Read the model definition and answer for the solid it produces. Units are mm, in the model's axes. Face numbers are marked on the shaded views. A direction names the side the tool comes from. Coordinates: 2 decimals unless noted, no trailing zeros. Write each loop counter-clockwise with the first axis right and the second up, starting at its lowest first coordinate (ties: lowest second). Pieces come first, ordered by that corner, then holes. Notation, with made-up numbers: (77, -3) - (113, -3) arc R24 ccw to (113, 29) - close; hole circle Ø9 at (85.25, -38). An arc over 180 degrees is marked (long way). Use a Markdown table: item, result.
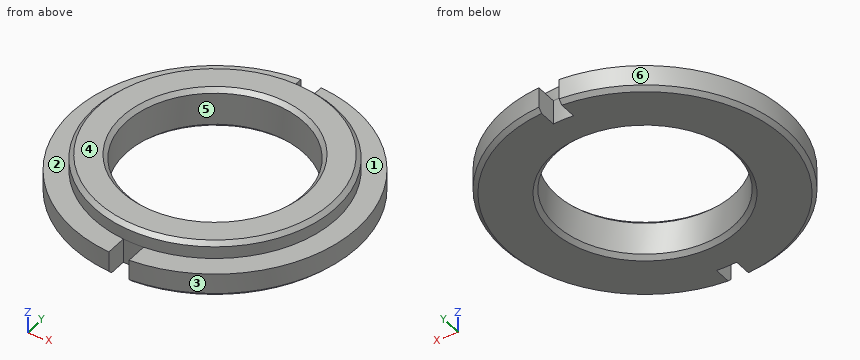
from build123d import *

# Parameters (mm, degrees)
SKETCH1_R           = 17.65
SKETCH1_R_2         = 11
BOSS_EXTRUDE1_DEPTH = 5
SKETCH2_R           = 17.65
SKETCH2_R_2         = 15
CUT_EXTRUDE1_DEPTH  = 2
CUT_EXTRUDE3_REACH  = 5
CHAMFER1_SIZE       = 0.5


with BuildPart() as part:
    # Sketch1 → Boss-Extrude1 (new body)
    with BuildSketch(Plane.XY):
        Circle(SKETCH1_R)
        Circle(SKETCH1_R_2, mode=Mode.SUBTRACT)
    extrude(amount=BOSS_EXTRUDE1_DEPTH)

    # Sketch2 → Cut-Extrude1 (cut)
    with BuildSketch(Plane.XY.offset(5)):
        Circle(SKETCH2_R)
        Circle(SKETCH2_R_2, mode=Mode.SUBTRACT)
    extrude(amount=-CUT_EXTRUDE1_DEPTH, mode=Mode.SUBTRACT)

    # Sketch3 → Cut-Extrude3 (cut, up to next)
    with BuildSketch(Plane.XY.offset(3), mode=Mode.PRIVATE) as cut_extrude3_sk1:
        with BuildLine():
            Line((1.25, 17.605680901), (1.25, 14.947825929))
            ThreePointArc((1.25, 14.947825929), (0, 15), (-1.25, 14.947825929))
            Line((-1.25, 14.947825929), (-1.25, 17.605680901))
            ThreePointArc((-1.25, 17.605680901), (0, 17.65), (1.25, 17.605680901))
        make_face()
    cut_extrude3_tool1 = extrude(cut_extrude3_sk1.sketch, amount=-CUT_EXTRUDE3_REACH, mode=Mode.PRIVATE) & part.part
    add(cut_extrude3_tool1.solids().sort_by_distance((0, 16.308915, 3))[0], mode=Mode.SUBTRACT)
    # Sketch3 → Cut-Extrude3 (cut, up to next)
    with BuildSketch(Plane.XY.offset(3), mode=Mode.PRIVATE) as cut_extrude3_sk2:
        with BuildLine():
            Line((1.25, -14.947825929), (1.25, -17.605680901))
            ThreePointArc((1.25, -17.605680901), (0, -17.65), (-1.25, -17.605680901))
            Line((-1.25, -17.605680901), (-1.25, -14.947825929))
            ThreePointArc((-1.25, -14.947825929), (0, -15), (1.25, -14.947825929))
        make_face()
    cut_extrude3_tool2 = extrude(cut_extrude3_sk2.sketch, amount=-CUT_EXTRUDE3_REACH, mode=Mode.PRIVATE) & part.part
    add(cut_extrude3_tool2.solids().sort_by_distance((0, -16.308915, 3))[0], mode=Mode.SUBTRACT)

    # Chamfer1
    chamfer1_edges = [part.edges().sort_by_distance(p)[0] for p in [
        (-15, 0, 5),
        (-17.65, 0, 0),
        (17.65, 0, 0),
        (-11, 0, 0),
        (-11, 0, 5),
    ]]
    chamfer(chamfer1_edges, length=CHAMFER1_SIZE)


solid = part.part
(1) The mould has two halves that part along Y. Classify the marked faces 4, 5 and 6: pulls with the +Y half, pulls with the -Y half, needs draft (parallel to the pull), parting line crosses it, or undercut.
Report:
| item | result |
|---|---|
| face 4 | needs draft |
| face 5 | undercut |
| face 6 | parting line crosses it |
(2) Each of these flat-tipped pins is pushed along its axis until it touches: P1, Ø3, axis at y = -3.5, z = 3.5, coming from the -X side; P2, Ø2, axis at x = 13, z = 1, coming from the -Y side; P3, Ø5, axis at x = 8.5, y = -6.5, coming from the +Z side; P4, Ø2, axis at y = 16.5, z = 1, coming from the -X side. Where does it stop, or does it pass through?
Report:
| item | result |
|---|---|
| P1 | stops at x = -17.53 |
| P2 | stops at y = -12.94 |
| P3 | stops at z = 5 |
| P4 | stops at x = -8.44 |
(3) A cutting plane is placed at A-A, the plane y = 0. Write down the section's boundary in (x, z).
Report:
| item | result |
|---|---|
| outline | (-17.65, 0.5) - (-17.15, 0) - (-11.5, 0) - (-11, 0.5) - (-11, 4.5) - (-11.5, 5) - (-14.5, 5) - (-15, 4.5) - (-15, 3) - (-17.65, 3) - close; (11, 0.5) - (11.5, 0) - (17.15, 0) - (17.65, 0.5) - (17.65, 3) - (15, 3) - (15, 4.5) - (14.5, 5) - (11.5, 5) - (11, 4.5) - close |
(4) Straight lines are drawn through the part: L1, parallel to Y at x = 0, z = 3.45; L2, parallel to X at y = -8, z = 4.8; L3, parallel to X at y = 2.5, z = 0.6. For each, find the intervals that lie inside material, in ascending order.
Report:
| item | result |
|---|---|
| L1 | y = -15 to -11, 11 to 15 |
| L2 | x = -12.33 to -7.98, 7.98 to 12.33 |
| L3 | x = -17.47 to -10.71, 10.71 to 17.47 |
(5) A cutting plane is placed at B-B, the plane x = 0. Write down the section's boundary in (y, z).
Report:
| item | result |
|---|---|
| outline | (-15, 0) - (-11.5, 0) - (-11, 0.5) - (-11, 4.5) - (-11.5, 5) - (-14.5, 5) - (-15, 4.5) - close; (11, 0.5) - (11.5, 0) - (15, 0) - (15, 4.5) - (14.5, 5) - (11.5, 5) - (11, 4.5) - close |
(6) For the marked faces 1, 2 and 3, determine the directions among +Z, -Z, +X, -X, +Y, -Y from which every point of the face is accessible in a straight line to the end or side of a thin tool.
Report:
| item | result |
|---|---|
| face 1 | +Z, +X |
| face 2 | +Z, -X |
| face 3 | +Z, -Z, +X |
